Could you check a few things on this drawing? It's one solid part, dimensions in mm from its lowest x, y, z. Give positions to 0.01 mm unless a question says otherwise; leave off trailing zeros. Order: outer loops, then holes, each group sorted by start corner. A loop starts at its lowest first (then second) coordinate and runs counter-clockwise, first axis right, second up. Notation, with made-up numbers: (-21.75, -34.75) - (-0.75, -34.75) arc R17 cw to (-0.75, -3.75) - close; hole circle Ø4 at (-14.75, 0). An arc over 180 degrees is marked (long way). Answer as CSV lines item,"result".
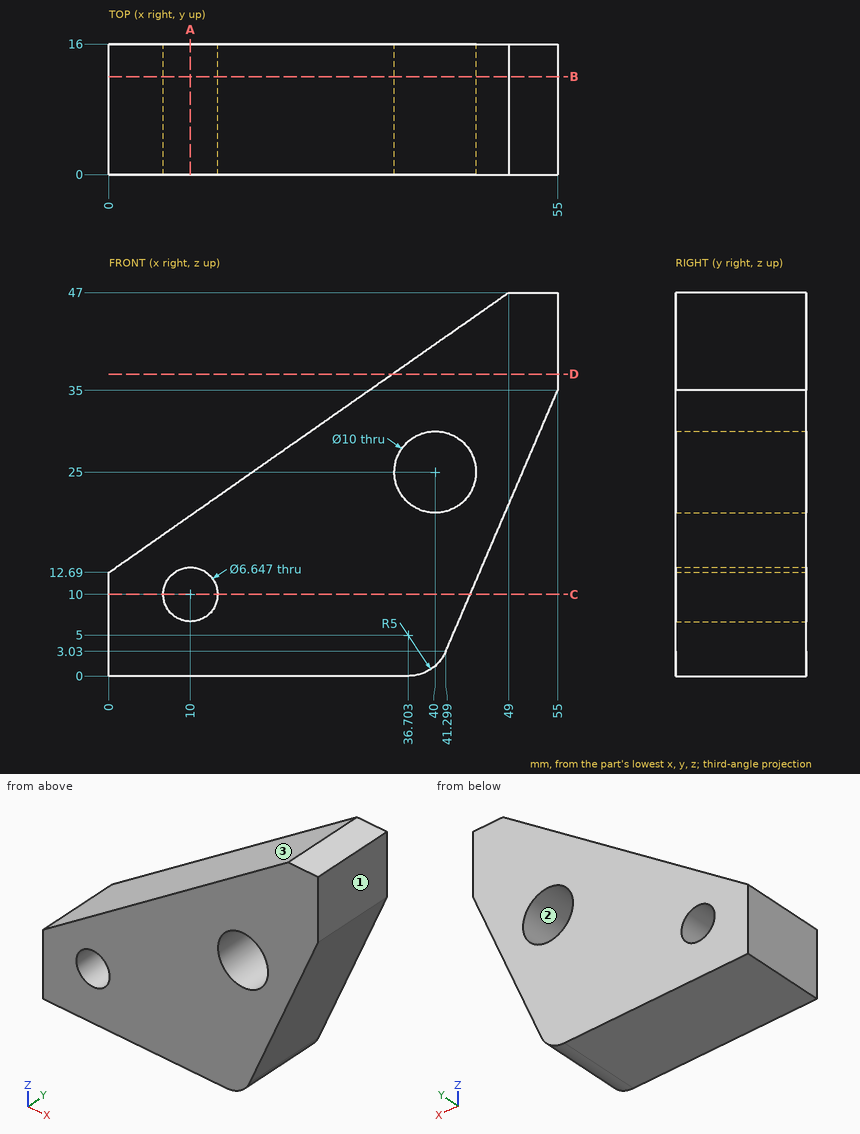
1) If we mould it in two halves opening along Z, with no side actions, what happens to the marked faces 1, 2 and 3? For each: +Z half, -Z half, draft (parallel to the pull), parting line (faces both ways), or undercut.
Answer block:
face 1,"draft"
face 2,"undercut"
face 3,"+Z half"
2) I want a section at D-D on z = 37. Write out the boundary of the cut face in (x, y).
Answer block:
outline,"(34.72, 0) - (55, 0) - (55, 16) - (34.72, 16) - close"
3) I need wall thicknesses on line 1 along Z through (x, y) = (10, 9.25) (1 decimal); line 2 along X through (y, z) = (7, 25) (1 decimal); line 3 along Z through (x, y) = (40, 4). Which ranges of each line are inside material? Lowest first, please. Write a range as [from, to].
Answer block:
line 1,"[0, 6.7], [13.3, 19.7]"
line 2,"[17.6, 35], [45, 50.7]"
line 3,"[1.24, 20], [30, 40.7]"
4) I want a section at B-B on y = 12. Write out the boundary of the cut face in (x, z).
Answer block:
outline,"(0, 0) - (36.7, 0) arc R5 ccw to (41.3, 3.03) - (55, 35) - (55, 47) - (49, 47) - (0, 12.69) - close; hole circle Ø6.65 at (10, 10); hole circle Ø10 at (40, 25)"
5) I want a section at A-A on x = 10. Write out the boundary of the cut face in (y, z), plus the area to 3 significant figures.
Answer block:
outline,"(0, 0) - (16, 0) - (16, 6.68) - (0, 6.68) - close; (0, 13.32) - (16, 13.32) - (16, 19.69) - (0, 19.69) - close"
area,"209 mm2"
6) I'm going to push flat-ended pins straight in: P1, Ø1, axis at y = 8.5, z = 32, coming from the -X side (1 decimal); P2, Ø3, axis at y = 7.5, z = 31, coming from the +X side; P3, Ø1, axis at y = 5.5, z = 42, coming from the -X side (1 decimal); P4, Ø6, axis at x = 10, z = 10, coming from the +Y side. Where does each tip first touch, or does it pass through?
Answer block:
P1,"x = 26.9"
P2,"x = 53.93"
P3,"x = 41.1"
P4,"through"
7) I want a section at C-C on z = 10. Write out the boundary of the cut face in (x, y) (1 decimal), plus the area to 3 significant figures.
Answer block:
outline,"(0, 0) - (6.7, 0) - (6.7, 16) - (0, 16) - close; (13.3, 0) - (44.3, 0) - (44.3, 16) - (13.3, 16) - close"
area,"602 mm2"
